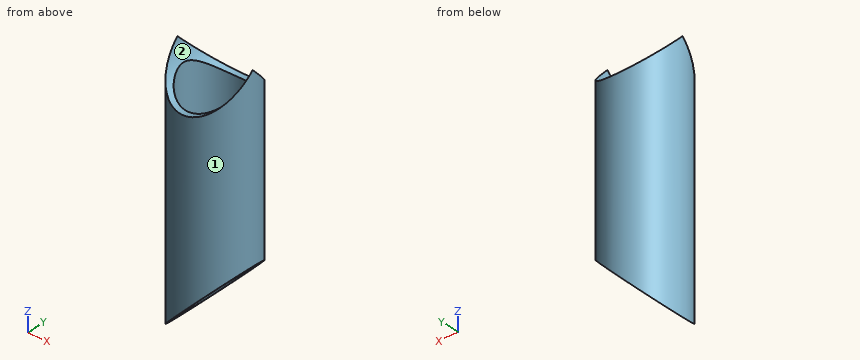
from build123d import *

# Parameters (mm, degrees)
F0_R     = 15
F0_R_2   = 12.5
F1_DEPTH = 49.9264
F2_R     = 15
F3_DEPTH = 25
F5_DEPTH = 15
F6_DEPTH = 25


with BuildPart() as f1:
    # F0 (on Top) → F1 (new body, symmetric)
    with BuildSketch(Plane.XY):
        Circle(F0_R)
        Circle(F0_R_2, mode=Mode.SUBTRACT)
    extrude(amount=F1_DEPTH, both=True)

    # F2 (on Front) → F3 (cut, symmetric)
    with BuildSketch(Plane.XZ):
        with Locations((0, 49.9264)):
            Circle(F2_R)
    extrude(amount=F3_DEPTH, both=True, mode=Mode.SUBTRACT)

    # F4 (on Front) → F5 (cut, symmetric)
    with BuildSketch(Plane.XZ):
        Polygon((15, -19.9264), (-15, -49.9264), (15, -49.9264), align=None)
    extrude(amount=F5_DEPTH, both=True, mode=Mode.SUBTRACT)

    # F4 (on Front) → F6 (cut, symmetric)
    with BuildSketch(Plane.XZ):
        Polygon((15, -19.9264), (-15, -49.9264), (15, -49.9264), align=None)
    extrude(amount=F6_DEPTH, both=True, mode=Mode.SUBTRACT)


solid = f1.part
Could you check a few things on this model? Use its own coordinates, in mm. Face numbers are marked on the shaded views. Give positions to 0.01 mm unless a question says otherwise; leave off trailing zeros. Order: outer loops, then holes, each group sorted by start corner. A loop starts at its lowest first (then second) coordinate and runs counter-clockwise, first axis right, second up.
Item 1: If we section it at A-A, the plane y = 0: Write out the boundary of the cut face in (x, z), plus the area to 3 significant figures.
Item 2: If we section it at D-D, the plane z = -32.5: Write out the boundary of the cut face in (x, y).
Item 3: If we mould it in two halves opening along X, with no side actions, what happens to the marked faces 1 and 2? For each: pulls with the +X half, pulls with the -X half, needs draft (parallel to the pull), parting line crosses it, or undercut.
Item 4: If we section it at C-C, the plane z = -9: Write out the boundary of the cut face in (x, y).
Item 5: I'm going to push flat-ended pins straight in: pin 1 (3 mm diameter, centred on y = 2.5, z = -25.5, fed in from +X); pin 2 (10 mm diameter, centred on y = -9.5, z = -36, fed in from -X); pin 3 (6 mm diameter, centred on x = -10, z = 34.5, fed in from +Y). Where does each tip first touch, or does it pass through?
Item 6: I need wall thicknesses on line 1 (Y direction, x = 0, z = -8); line 2 (X direction, y = 10.5, z = -16.5); line 3 (X direction, y = 9, z = 3.5). Which ranges of each line are inside material? Lowest first, please.
Item 7: If we section it at B-B, the plane x = 0: Write out the boundary of the cut face in (y, z).
Values:
1. outline: (-15, -49.93) - (-12.5, -47.43) - (-12.5, 41.63) arc R15 cw to (-15, 49.93) - close; (12.5, -22.43) - (15, -19.93) - (15, 49.93) arc R15 cw to (12.5, 41.63) - close
1. area: 396 mm2
2. outline: (2.43, -14.8) - (2.43, -12.26) arc R12.5 cw (long way) to (2.43, 12.26) - (2.43, 14.8) arc R15 ccw (long way) to start
3. face 1: parting line crosses it
3. face 2: undercut
4. outline: circle Ø30 at (0, 0); hole circle Ø25 at (0, 0)
5. pin 1: stops at x = -11.84
5. pin 2: stops at x = -14.31
5. pin 3: stops at y = 13.27
6. line 1: y = -15 to -12.5, 12.5 to 15
6. line 2: x = -10.71 to -6.78, 6.78 to 10.71
6. line 3: x = -12 to -8.67, 8.67 to 12
7. outline: (-15, -34.93) - (-12.5, -34.93) - (-12.5, 34.93) - (-15, 34.93) - close; (12.5, -34.93) - (15, -34.93) - (15, 34.93) - (12.5, 34.93) - close
